```python
from build123d import *

# Parameters (mm, degrees)
IZIM1_W                     = 70
IZIM1_H                     = 20
Y_KSEKLIK_EKSTR_ZYON1_DEPTH = 4.6
IZIM2_R                     = 1.5
KES_EKSTR_ZYON1_DEPTH       = 4.6
IZIM3_R                     = 3
KES_EKSTR_ZYON2_DEPTH       = 3


with BuildPart() as part:
    # Çizim1 → Yükseklik-Ekstrüzyon1 (new body)
    with BuildSketch(Plane(origin=(0, 0, 0), x_dir=(1, 0, 0), z_dir=(0, 1, 0))):
        with Locations((35, 10)):
            Rectangle(IZIM1_W, IZIM1_H)
    extrude(amount=Y_KSEKLIK_EKSTR_ZYON1_DEPTH)

    # Çizim2 → Kes-Ekstrüzyon1 (cut)
    with BuildSketch(Plane.XZ):
        with Locations(Location((58.5, -10, 0), (0, 0, 270))):
            Circle(IZIM2_R)
        with Locations(Location((11.5, -10, 0), (0, 0, 270))):
            Circle(IZIM2_R)
    extrude(amount=-KES_EKSTR_ZYON1_DEPTH, mode=Mode.SUBTRACT)

    # Çizim3 → Kes-Ekstrüzyon2 (cut)
    with BuildSketch(Plane.XZ):
        with Locations(Location((11.5, -10, 0), (0, 0, 270))):
            Circle(IZIM3_R)
        with Locations(Location((58.5, -10, 0), (0, 0, 270))):
            Circle(IZIM3_R)
    extrude(amount=-KES_EKSTR_ZYON2_DEPTH, mode=Mode.SUBTRACT)


solid = part.part
```
CAD build for the part. Positions are in the model's coordinates, mm. A direction names the side the tool comes from. Round coordinates to 2 decimals unless told otherwise and drop trailing zeros. Order: outer loops, then holes, each group sorted by start corner. A loop starts at its lowest first (then second) coordinate and runs counter-clockwise, first axis right, second up.
Item 1: Pin check, flat tip, straight feed: pin 1 (5 mm diameter, centred on x = 58.5, z = -10, fed in from -Y). Stop position of the tip, or through.
Item 2: Probe line 1 along X through (y, z) = (1.5, -10); line 2 along X through (y, z) = (3.85, -10); line 3 along Z through (x, y) = (57, 1.6). List the from-to ranges inside material, lowest first.
Item 3: Mould opens along X. For faces 3 (the face through (61.03, 1.48, -11.61)), 4 (the face through (35, 0, -10)), 5 (the face through (70, 2, -10)) say: pulls with the +X half, pulls with the -X half, needs draft (parallel to the pull), parting line crosses it, or undercut.
Item 4: Saw through at A-A on x = 58.5. Write the cut outline in (y, z), then the cut area to 3 significant figures.
Item 5: Saw through at C-C on y = 1.2. Write the cut outline in (x, z), then the cut area to 3 significant figures.
Item 6: Saw through at B-B on z = -10. Write the cut outline in (x, y), then the cut area to 3 significant figures.
Item 7: Tool access for faces 1 (the face through (10.35, 1.48, -12.77)), 2 (the face through (60, 4, -10)): list every direction of +Z, -Z, +X, -X, +Y, -Y with a clear straight run to the whole face (end or side of a thin tool).
Reported:
1. pin 1: stops at y = 3
2. line 1: x = 0 to 8.5, 14.5 to 55.5, 61.5 to 70
2. line 2: x = 0 to 10, 13 to 57, 60 to 70
2. line 3: z = -20 to -12.6, -7.4 to 0
3. face 3: undercut
3. face 4: needs draft
3. face 5: pulls with the +X half
4. outline: (0, -20) - (4.6, -20) - (4.6, -11.5) - (3, -11.5) - (3, -13) - (0, -13) - close; (0, -7) - (3, -7) - (3, -8.5) - (4.6, -8.5) - (4.6, 0) - (0, 0) - close
4. area: 69.2 mm2
5. outline: (0, -20) - (70, -20) - (70, 0) - (0, 0) - close; hole circle Ø6 at (11.5, -10); hole circle Ø6 at (58.5, -10)
5. area: 1,340 mm2
6. outline: (0, 0) - (8.5, 0) - (8.5, 3) - (10, 3) - (10, 4.6) - (0, 4.6) - close; (13, 3) - (14.5, 3) - (14.5, 0) - (55.5, 0) - (55.5, 3) - (57, 3) - (57, 4.6) - (13, 4.6) - close; (60, 3) - (61.5, 3) - (61.5, 0) - (70, 0) - (70, 4.6) - (60, 4.6) - close
6. area: 276 mm2
7. face 1: -Y
7. face 2: +Y, -Y
